Read the model definition and answer for the solid it produces. Units are mm, in the model's axes. A direction names the side the tool comes from. Coordinates: 2 decimals unless noted, no trailing zeros. Order: outer loops, then holes, each group sorted by start corner. A loop starts at its lowest first (then second) coordinate and runs counter-clockwise, first axis right, second up. Notation, with made-up numbers: M 89.25,30 L 117.25,30 A10 ccw 117.25,45 Z; hole C -20.75,-22.75 d3. An arc over 180 degrees is marked long. Write each question's results on one line, items separated by ' | '.
```python
from build123d import *

# Parameters (mm, degrees)
SKETCH1_W           = 1695.45
SKETCH1_H           = 184.15
BOSS_EXTRUDE1_DEPTH = 38.1
SKETCH2_W           = 38.1
SKETCH2_H           = 95.25
BOSS_EXTRUDE3_DEPTH = 38.1
CHAMFER1_SIZE       = 2.54
CHAMFER2_SIZE       = 2.54
SKETCH3_R           = 19.05
CUT_EXTRUDE1_DEPTH  = 3.175


with BuildPart() as part:
    # Sketch1 → Boss-Extrude1 (new body)
    with BuildSketch(Plane(origin=(0, 0, 0), x_dir=(1, 0, 0), z_dir=(0, 1, 0))):
        with Locations((847.725, 92.075)):
            Rectangle(SKETCH1_W, SKETCH1_H)
        with BuildLine():
            Line((1181.2651, 135.56615), (1240.0153, 135.56615))
            ThreePointArc((1240.0153, 135.56615), (1252.7153, 122.86615), (1240.0153, 110.16615))
            Line((1240.0153, 110.16615), (1181.2651, 110.16615))
            ThreePointArc((1181.2651, 110.16615), (1168.5651, 122.86615), (1181.2651, 135.56615))
        make_face(mode=Mode.SUBTRACT)
        with BuildLine():
            Line((254, 110.31855), (312.7502, 110.31855))
            ThreePointArc((312.7502, 110.31855), (325.4502, 97.61855), (312.7502, 84.91855))
            Line((312.7502, 84.91855), (254, 84.91855))
            ThreePointArc((254, 84.91855), (241.3, 97.61855), (254, 110.31855))
        make_face(mode=Mode.SUBTRACT)
    extrude(amount=BOSS_EXTRUDE1_DEPTH)

    # Sketch2 → Boss-Extrude3 (add, through all)
    with BuildSketch(Plane(origin=(0, 38.1, 0), x_dir=(1, 0, 0), z_dir=(0, 1, 0))):
        with Locations((-19.05, 47.625)):
            Rectangle(SKETCH2_W, SKETCH2_H)
    extrude(amount=-BOSS_EXTRUDE3_DEPTH)

    # Chamfer1
    chamfer1_edges = [part.edges().sort_by_distance(p)[0] for p in [
        (1695.45, 38.1, -92.075),
        (1252.7153, 38.1, -122.86615),
        (847.725, 38.1, -184.15),
        (1210.6402, 38.1, -135.56615),
        (1168.5651, 38.1, -122.86615),
        (1210.6402, 38.1, -110.16615),
        (325.4502, 38.1, -97.61855),
        (283.3751, 38.1, -110.31855),
        (241.3, 38.1, -97.61855),
        (283.3751, 38.1, -84.91855),
        (-19.05, 38.1, -95.25),
        (-38.1, 38.1, -47.625),
        (0, 38.1, -139.7),
        (828.675, 38.1, 0),
    ]]
    chamfer(chamfer1_edges, length=CHAMFER1_SIZE)

    # Chamfer2
    chamfer2_edges = [part.edges().sort_by_distance(p)[0] for p in [
        (1252.7153, 0, -122.86615),
        (1210.6402, 0, -135.56615),
        (1168.5651, 0, -122.86615),
        (1210.6402, 0, -110.16615),
        (325.4502, 0, -97.61855),
        (283.3751, 0, -110.31855),
        (241.3, 0, -97.61855),
        (283.3751, 0, -84.91855),
        (-38.1, 0, -47.625),
        (-19.05, 0, -95.25),
        (847.725, 0, -184.15),
        (1695.45, 0, -92.075),
        (828.675, 0, 0),
        (0, 0, -139.7),
    ]]
    chamfer(chamfer2_edges, length=CHAMFER2_SIZE)

    # Sketch3 → Cut-Extrude1 (cut)
    with BuildSketch(Plane(origin=(0, 38.1, 0), x_dir=(1, 0, 0), z_dir=(0, 1, 0))):
        with Locations((1210.6402, 122.86615)):
            Circle(SKETCH3_R)
        with Locations((283.3751, 97.61855)):
            Circle(SKETCH3_R)
    extrude(amount=-CUT_EXTRUDE1_DEPTH, mode=Mode.SUBTRACT)


solid = part.part
```
(1) Straight lines are drawn through the part: line 1 (X direction, y = 4.5, z = -98); line 2 (X direction, y = 14.5, z = -125); line 3 (X direction, y = 18.5, z = -140.5). For each, find the intervals that lie inside material, in ascending order.
Conclusion:
line 1: 0 to 241.31, 325.44 to 1695.45 | line 2: 0 to 1168.75, 1252.53 to 1695.45 | line 3: 0 to 1695.45
(2) For faces 1 (the flat face through (0, 19, -139)), 2 (the flat face through (1211, 19, -110.166)), 3 (the flat face through (1695.45, 19, -91)), determine the directions among +Z, -Z, +X, -X, +Y, -Y from which every point of the face is accessible in a straight line to the end or side of a thin tool.
Conclusion:
face 1: -Z, -X, +Y, -Y | face 2: +Y, -Y | face 3: +Z, -Z, +X, +Y, -Y
(3) Given pin 1 (5 mm diameter, centred on y = 16, z = -124, fed in from -X); pin 2 (1.9 mm diameter, centred on x = 1208.5, z = -140, fed in from +Y) (3 decimals); pin 3 (10 mm diameter, centred on x = -22.5, y = 21, fed in from -Z), each flat-ended and moving along its own axis, determine where each tip first touches the part or whether it passes through.
Conclusion:
pin 1: x = 0 | pin 2: y = 34.925 | pin 3: z = -95.25
(4) The part is cut by section A-A, the plane y = 24. Write down the section's boundary in (x, z).
Conclusion:
outline: M -38.1,-95.25 L 0,-95.25 L 0,-184.15 L 1695.45,-184.15 L 1695.45,0 L -38.1,0 Z; hole M 254,-110.32 L 312.75,-110.32 A12.7 ccw 312.75,-84.92 L 254,-84.92 A12.7 ccw Z; hole M 1181.27,-135.57 L 1240.02,-135.57 A12.7 ccw 1240.02,-110.17 L 1181.27,-110.17 A12.7 ccw Z
(5) The mould has two halves that part along Z. Classify faces 4 (the flat face through (284, 19, -84.919)), 5 (the flat face through (817, 0, -93)), 6 (the flat face through (836, 19, -184.15)), 7 (the flat face through (283, 19, -110.319)): pulls with the +Z half, pulls with the -Z half, needs draft (parallel to the pull), parting line crosses it, or undercut.
Conclusion:
face 4: undercut | face 5: needs draft | face 6: pulls with the -Z half | face 7: undercut
